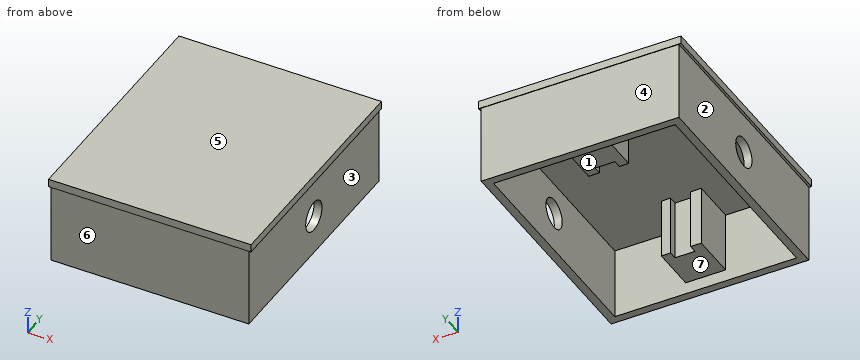
from build123d import *

# Parameters (mm, degrees)
F0_W     = 62.865
F0_H     = 25.4
F1_DEPTH = 76.2
F3_T     = -2.54
F4_W     = 64.389
F4_H     = 76.454
F5_DEPTH = 2.54
F2_R     = 4.7625
F6_DEPTH = 63.628
F8_DEPTH = 19.05


with BuildPart() as f1:
    # F0 (on Front) → F1 (new body)
    with BuildSketch(Plane.XZ):
        Rectangle(F0_W, F0_H)
    extrude(amount=F1_DEPTH)

    # F3
    f3_openings = [f1.faces().sort_by_distance(p)[0] for p in [
        (0, -38.1, -12.7),
    ]]
    offset(amount=F3_T, openings=f3_openings)

    # F4 (on face) → F5 (join)
    with BuildSketch(Plane.XY.offset(12.7)):
        with Locations((0, -38.1)):
            Rectangle(F4_W, F4_H)
    extrude(amount=F5_DEPTH)

    # F2 (on face) → F6 (cut, through all)
    with BuildSketch(Plane.YZ.offset(31.4325)):
        with Locations((-38.1, 0)):
            Circle(F2_R)
    extrude(amount=-F6_DEPTH, mode=Mode.SUBTRACT)

    # F7 (on face) → F8 (join)
    with BuildSketch(Plane(origin=(0, 0, 10.16), x_dir=(1, 0, 0), z_dir=(0, 0, -1))):
        Polygon((-2.976563, 61.9125), (3.373437, 61.9125), (3.373437, 59.27708), (6.35, 59.3725), (6.35, 61.9125), (6.35, 73.66), (0, 73.66), (-6.35, 73.66), (-6.35, 61.9125), (-6.35, 59.3725), (-2.976563, 59.3725), align=None)
        Polygon((2.976563, 16.8275), (2.976563, 14.2875), (-3.373437, 14.2875), (-3.373437, 16.8275), (-6.35, 16.8275), (-6.35, 14.2875), (-6.35, 2.54), (6.35, 2.54), (6.35, 14.2875), (6.35, 16.8275), align=None)
    extrude(amount=F8_DEPTH)


solid = f1.part
The model under review builds one solid part; all positions refer to its coordinate system, in mm. Face numbers are marked on the shaded views. A direction names the side the tool comes from. Coordinates: 2 decimals unless noted, no trailing zeros. Write each loop counter-clockwise with the first axis right and the second up, starting at its lowest first coordinate (ties: lowest second). Pieces come first, ordered by that corner, then holes. Notation, with made-up numbers: (80.5, 10) - (88.5, 10) arc R22 ccw to (88.5, 36) - close; hole circle Ø3 at (20.25, -25.5). An arc over 180 degrees is marked (long way). Answer as a JSON object with one key per item and string values. Group by question number.
1. Mouldability with a two-part tool opening along X and no side actions: class the marked faces 1, 2, 3 and 4 as pulls with the +X half, pulls with the -X half, needs draft (parallel to the pull), parting line crosses it, or undercut.
2. Add section B-B (y = -38.1). Give the boundary of the cut face in (x, z).
3. To check wall thickness, follow probe 1 along X at (y, z) = (-64, 9.75); probe 2 along Z at (x, y) = (30, -38); probe 3 along Y at (x, z) = (-24, -4.25). State the ranges of each line that lie inside material, in increasing order.
4. Add section D-D (y = -58). Give the boundary of the cut face in (x, z), plus the area to 3 significant figures.
5. Clearance check with flat-ended pins moving along their axes: pin 1 Ø12 at (x, z) = (-2, -7) entering from -Y; pin 2 Ø3 at (y, z) = (-16, -1) entering from +X; pin 3 Ø4 at (x, y) = (-3.5, -26.5) entering from -Z; pin 4 Ø4 at (y, z) = (-24.5, 12) entering from -X. State where each tip first meets the part, or that it passes through.
6. Machinability: for the marked faces 5, 6 and 7, which of the approach directions +Z, -Z, +X, -X, +Y, -Y give a long, thin tool a straight path to every point of the face, cutting with its end or side? Answer none if there is none.
7. Add section C-C (z = 8.25). Give the boundary of the cut face in (x, y), plus the area to 3 significant figures.
Findings:
{
 "1": {"face 1": "undercut", "face 2": "pulls with the -X half", "face 3": "pulls with the +X half", "face 4": "needs draft"},
 "2": {"outline": "(-32.19, 12.7) - (-31.43, 12.7) - (-31.43, 4.76) - (-28.89, 4.76) - (-28.89, 10.16) - (28.89, 10.16) - (28.89, 4.76) - (31.43, 4.76) - (31.43, 12.7) - (32.19, 12.7) - (32.19, 15.24) - (-32.19, 15.24) - close; (-31.43, -12.7) - (-28.89, -12.7) - (-28.89, -4.76) - (-31.43, -4.76) - close; (28.89, -12.7) - (31.43, -12.7) - (31.43, -4.76) - (28.89, -4.76) - close"},
 "3": {"probe 1": "-31.43 to -28.89, -6.35 to 6.35, 28.89 to 31.43", "probe 2": "-12.7 to -4.76, 4.76 to 15.24", "probe 3": "-76.2 to -73.66, -2.54 to 0"},
 "4": {"outline": "(-32.19, 12.7) - (-31.43, 12.7) - (-31.43, -12.7) - (-28.89, -12.7) - (-28.89, 10.16) - (28.89, 10.16) - (28.89, -12.7) - (31.43, -12.7) - (31.43, 12.7) - (32.19, 12.7) - (32.19, 15.24) - (-32.19, 15.24) - close", "area": "439 mm²"},
 "5": {"pin 1": "y = -76.2", "pin 2": "x = 31.43", "pin 3": "z = 10.16", "pin 4": "x = -32.19"},
 "6": {"face 5": "+Z, +X, -X, +Y, -Y", "face 6": "-Z, +X, -X, -Y", "face 7": "-Z"},
 "7": {"outline": "(-31.43, -76.2) - (31.43, -76.2) - (31.43, 0) - (-31.43, 0) - close; hole (-28.89, -73.66) - (-6.35, -73.66) - (-6.35, -59.37) - (-2.98, -59.37) - (-2.98, -61.91) - (3.37, -61.91) - (3.37, -59.28) - (6.35, -59.37) - (6.35, -73.66) - (28.89, -73.66) - (28.89, -2.54) - (6.35, -2.54) - (6.35, -16.83) - (2.98, -16.83) - (2.98, -14.29) - (-3.37, -14.29) - (-3.37, -16.83) - (-6.35, -16.83) - (-6.35, -2.54) - (-28.89, -2.54) - close", "area": "1,010 mm²"}
}
